from build123d import *

# Parameters (mm, degrees)
SKETCH1_R           = 27.5
BOSS_EXTRUDE1_DEPTH = 5
SKETCH2_R           = 25
SKETCH2_R_2         = 22.5
BOSS_EXTRUDE2_DEPTH = 5


with BuildPart() as part:
    # Sketch1 → Boss-Extrude1 (new body)
    with BuildSketch(Plane(origin=(0, 0, 0), x_dir=(1, 0, 0), z_dir=(0, 1, 0))):
        with Locations(Location((0, 0, 0), (0, 0, 270))):  # turned: the seam where the file's is
            Circle(SKETCH1_R)
    extrude(amount=BOSS_EXTRUDE1_DEPTH)

    # Sketch2 → Boss-Extrude2 (add)
    with BuildSketch(Plane(origin=(0, 5, 0), x_dir=(1, 0, 0), z_dir=(0, 1, 0))):
        with Locations(Location((0, 0, 0), (0, 0, 270))):  # turned: the seam where the file's is
            Circle(SKETCH2_R)
        with Locations(Location((0, 0, 0), (0, 0, 270))):  # turned: the seam where the file's is
            Circle(SKETCH2_R_2, mode=Mode.SUBTRACT)
    extrude(amount=BOSS_EXTRUDE2_DEPTH)


solid = part.part
Design review of the part built by this model. Coordinates are the model's own, in mm. A direction names the side the tool comes from. Give positions to 0.01 mm unless a question says otherwise; leave off trailing zeros. Loops run counter-clockwise (first coordinate to the right, second up) from the corner with the lowest first, then second, coordinate; pieces in that order, holes last. Notation, with made-up numbers: M -18.75,46.25 L 10.25,46.25 A25 ccw 10.25,75.25 Z; hole C 65,38 d1. An arc over 180 degrees is marked long. Answer as a JSON object with one key per item and string values.
Item 1: We need section C-C (y = 2.5). State the section outline as (x, z) points.
Output values:
{"outline": "C 0,0 d55"}
Item 2: Machinability: for faces 1 (the face through (0, 0, 0)), 2 (the face through (7.509, 7.465, 23.846)), which of the approach directions +Z, -Z, +X, -X, +Y, -Y give a long, thin tool a straight path to every point of the face, cutting with its end or side? Answer none if there is none.
Output values:
{"face 1": "+Z, -Z, +X, -X, -Y", "face 2": "+Y"}
Item 3: We need section A-A (z = 0). State the section outline as (x, y) points.
Output values:
{"outline": "M -27.5,0 L 27.5,0 L 27.5,5 L 25,5 L 25,10 L 22.5,10 L 22.5,5 L -22.5,5 L -22.5,10 L -25,10 L -25,5 L -27.5,5 Z"}
Item 4: For P1, Ø22.5, axis at x = 2.5, z = 5, coming from the +Y side; P2, Ø5, axis at y = 3.5, z = 5.5, coming from the +X side; P3, Ø2, axis at y = 4.5, z = 5, coming from the +X side, all flat-tipped, find the tip position at first contact; note any pin that passes through.
Output values:
{"P1": "stops at y = 5", "P2": "stops at x = 27.34", "P3": "stops at x = 27.21"}
Item 5: We need section B-B (x = 4). State the section outline as (y, z) points.
Output values:
{"outline": "M 0,-27.21 L 5,-27.21 L 5,-24.68 L 10,-24.68 L 10,-22.14 L 5,-22.14 L 5,22.14 L 10,22.14 L 10,24.68 L 5,24.68 L 5,27.21 L 0,27.21 Z"}
Item 6: Mouldability with a two-part tool opening along X and no side actions: class faces 3 (the face through (-24.397, 2.465, 12.69)), 4 (the face through (-22.3, 5, 12.1)), 5 (the face through (0, 5, 0)) as pulls with the +X half, pulls with the -X half, needs draft (parallel to the pull), parting line crosses it, or undercut.
Output values:
{"face 3": "parting line crosses it", "face 4": "needs draft", "face 5": "undercut"}
Item 7: Wall thickness on line 1 along X through (y, z) = (7.95, 0); line 2 along Y through (x, z) = (-13, -3); line 3 along Z through (x, y) = (15.5, 6.25): over which ranges is each line inside the solid? List them lowest first.
Output values:
{"line 1": "x = -25 to -22.5, 22.5 to 25", "line 2": "y = 0 to 5", "line 3": "z = -19.62 to -16.31, 16.31 to 19.62"}
